from build123d import *

# Parameters (mm, degrees)
F0_W     = 58.74
F0_H     = 42.7
F1_DEPTH = 14.08
F2_R     = 6
F3_W     = 37.578944
F3_H     = 25.973686
F4_DEPTH = 7.3
F5_SIZE  = 5


with BuildPart() as f1:
    # F0 (on Top) → F1 (new body)
    with BuildSketch(Plane.XY):
        Rectangle(F0_W, F0_H)
    extrude(amount=F1_DEPTH)

    # F2
    f2_edges = [f1.edges().sort_by_distance(p)[0] for p in [
        (0, -21.35, 0),
        (29.37, 0, 0),
        (0, 21.35, 0),
        (-29.37, 0, 0),
        (29.37, -21.35, 7.04),
        (29.37, 21.35, 7.04),
        (-29.37, 21.35, 7.04),
        (-29.37, -21.35, 7.04),
    ]]
    fillet(f2_edges, radius=F2_R)

    # F3 (on face) → F4 (cut)
    with BuildSketch(Plane.XY.offset(14.08)):
        Rectangle(F3_W, F3_H)
    extrude(amount=-F4_DEPTH, mode=Mode.SUBTRACT)

    # F5
    f5_edges = [f1.edges().sort_by_distance(p)[0] for p in [
        (-18.789472, -12.986843, 10.43),
    ]]
    chamfer(f5_edges, length=F5_SIZE)


solid = f1.part
Can you work these out from the model? Positions are in its coordinate system, mm. A direction names the side the tool comes from. Round coordinates to 2 decimals unless told otherwise and drop trailing zeros. Write each loop counter-clockwise with the first axis right and the second up, starting at its lowest first coordinate (ties: lowest second). Pieces come first, ordered by that corner, then holes. Notation, with made-up numbers: M 50.25,87 L 106.25,87 A11 cw 106.25,95 Z; hole C -30,-9.5 d7. An arc over 180 degrees is marked long. Use a Markdown table: item, result.
Item 1: I want a section at B-B (y = 11). List the corners of the cut face in (x, z) for me.
Found:
| item | result |
|---|---|
| outline | M -29.37,6 A6 ccw -23.37,0 L 23.37,0 A6 ccw 29.37,6 L 29.37,14.08 L 18.79,14.08 L 18.79,6.78 L -18.79,6.78 L -18.79,14.08 L -29.37,14.08 Z |
Item 2: For pin 1 Ø1 at (y, z) = (15.5, 2) entering from +X; pin 2 Ø2 at (y, z) = (2.5, 2.5) entering from +X; pin 3 Ø1 at (x, z) = (-16, 4.5) entering from +Y, each with a flat end and sliding along its axis, tell me the tip position at first contact or that it passes through.
Found:
| item | result |
|---|---|
| pin 1 | stops at x = 28.24 |
| pin 2 | stops at x = 28.82 |
| pin 3 | stops at y = 21.27 |
Item 3: I want a section at A-A (z = 9). List the corners of the cut face in (x, y) for me.
Found:
| item | result |
|---|---|
| outline | M -29.37,-15.35 A6 ccw -23.37,-21.35 L 23.37,-21.35 A6 ccw 29.37,-15.35 L 29.37,15.35 A6 ccw 23.37,21.35 L -23.37,21.35 A6 ccw -29.37,15.35 Z; hole M -18.79,-7.99 L -13.79,-12.99 L 18.79,-12.99 L 18.79,12.99 L -18.79,12.99 Z |
Item 4: I want a section at D-D (z = 1.5). List the corners of the cut face in (x, y) for me.
Found:
| item | result |
|---|---|
| outline | M -27.34,-15.35 A3.97 ccw -23.37,-19.32 L 23.37,-19.32 A3.97 ccw 27.34,-15.35 L 27.34,15.35 A3.97 ccw 23.37,19.32 L -23.37,19.32 A3.97 ccw -27.34,15.35 Z |
Item 5: I want a section at C-C (x = 12). List the corners of the cut face in (y, z) for me.
Found:
| item | result |
|---|---|
| outline | M -21.35,6 A6 ccw -15.35,0 L 15.35,0 A6 ccw 21.35,6 L 21.35,14.08 L 12.99,14.08 L 12.99,6.78 L -12.99,6.78 L -12.99,14.08 L -21.35,14.08 Z |
Item 6: If I drill on line 1 along X through (y, z) = (7.5, 10.25); line 2 along Z through (x, y) = (-15.5, -1); line 3 along Z through (x, y) = (13, -15.5), over which ranges is the centre line in solid material (lowest first)? Write a range as [from, to].
Found:
| item | result |
|---|---|
| line 1 | x = [-29.37, -18.79], [18.79, 29.37] |
| line 2 | z = [0, 6.78] |
| line 3 | z = [0, 14.08] |
Item 7: We'd pull the mould along Y, two halves only. Please class faces 3 (the face through (-27.659, 19.546, 10.097)), 4 (the face through (0, 12.987, 10)), 5 (the face through (27.566, -19.639, 10.097)): released by +Y, released by -Y, zero draft, split by the parting line, or undercut.
Found:
| item | result |
|---|---|
| face 3 | released by +Y |
| face 4 | undercut |
| face 5 | released by -Y |
Item 8: Which directions (+Z, -Z, +X, -X, +Y, -Y) give clear straight access to the entire face, cutting with the end or side of a thin tool? Please do faces 1 (the face through (-27.659, -19.546, 10.097)), 2 (the face through (0, 0, 6.78)).
Found:
| item | result |
|---|---|
| face 1 | +Z, -Z, -X, -Y |
| face 2 | +Z |
